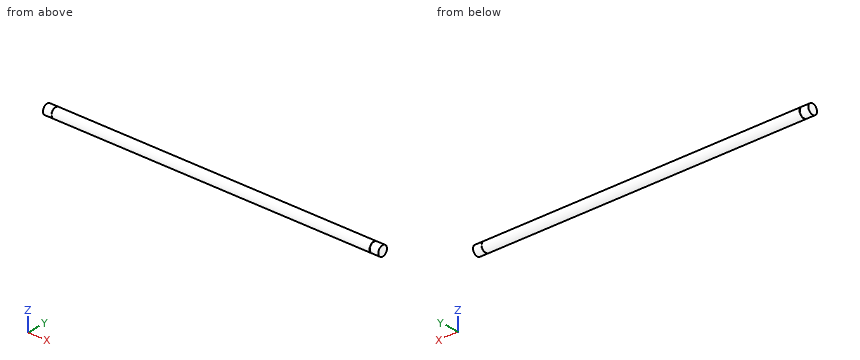
from build123d import *

# Parameters (mm, degrees)
F0_R     = 17.5
F1_DEPTH = 1200
F2_W     = 1.6
F2_H     = 1


with BuildPart() as f1:
    # F0 (on Right) → F1 (new body)
    with BuildSketch(Plane.YZ):
        Circle(F0_R)
    extrude(amount=-F1_DEPTH)

    # F2 (on Front) → F3 (revolve, cut)
    with BuildSketch(Plane.XZ):
        with Locations((-30.8, 17)):
            Rectangle(F2_W, F2_H)
        with Locations((-1169.2, 17)):
            Rectangle(F2_W, F2_H)
    revolve(axis=Axis((-600, 0, 0), (-1, 0, 0)), mode=Mode.SUBTRACT)


solid = f1.part
Design review of the part built by this model. Coordinates are the model's own, in mm. Coordinates: 2 decimals unless noted, no trailing zeros. Loops run counter-clockwise (first coordinate to the right, second up) from the corner with the lowest first, then second, coordinate; pieces in that order, holes last.
Item 1: Wall thickness on L1, parallel to Y at x = -892, z = 0.5; L2, parallel to Y at x = -568.5, z = 6: over which ranges is each line inside the solid? List them lowest first.
Completed:
L1: y = -17.49 to 17.49
L2: y = -16.44 to 16.44
Item 2: Clearance check with flat-ended pins moving along their axes: pin 1 (12 mm diameter, centred on y = 9, z = 8.5, fed in from +X); pin 2 (2 mm diameter, centred on x = -392.5, y = 5.5, fed in from +Z); pin 3 (8 mm diameter, centred on x = -211.5, z = 13, fed in from +Y); pin 4 (2 mm diameter, centred on x = -182.5, y = 7, fed in from +Z). State where each tip first meets the part, or that it passes through.
Completed:
pin 1: stops at x = 0
pin 2: stops at z = 16.91
pin 3: stops at y = 15.01
pin 4: stops at z = 16.44
Item 3: Add section A-A (y = -8.5). Write out the cut boundary in (x, z), and give its area (3 significant figures).
Completed:
outline: (-1200, -15.3) - (-1170, -15.3) - (-1170, -14.14) - (-1168.4, -14.14) - (-1168.4, -15.3) - (-31.6, -15.3) - (-31.6, -14.14) - (-30, -14.14) - (-30, -15.3) - (0, -15.3) - (0, 15.3) - (-30, 15.3) - (-30, 14.14) - (-31.6, 14.14) - (-31.6, 15.3) - (-1168.4, 15.3) - (-1168.4, 14.14) - (-1170, 14.14) - (-1170, 15.3) - (-1200, 15.3) - close
area: 36,700 mm2
Item 4: Add section C-C (x = -729.5). Write out the cut boundary in (y, z), and give its area (3 significant figures).
Completed:
outline: circle Ø35 at (0, 0)
area: 962 mm2
Item 5: Add section B-B (z = 6). Write out the cut boundary in (x, y).
Completed:
outline: (-1200, -16.44) - (-1170, -16.44) - (-1170, -15.37) - (-1168.4, -15.37) - (-1168.4, -16.44) - (-31.6, -16.44) - (-31.6, -15.37) - (-30, -15.37) - (-30, -16.44) - (0, -16.44) - (0, 16.44) - (-30, 16.44) - (-30, 15.37) - (-31.6, 15.37) - (-31.6, 16.44) - (-1168.4, 16.44) - (-1168.4, 15.37) - (-1170, 15.37) - (-1170, 16.44) - (-1200, 16.44) - close
